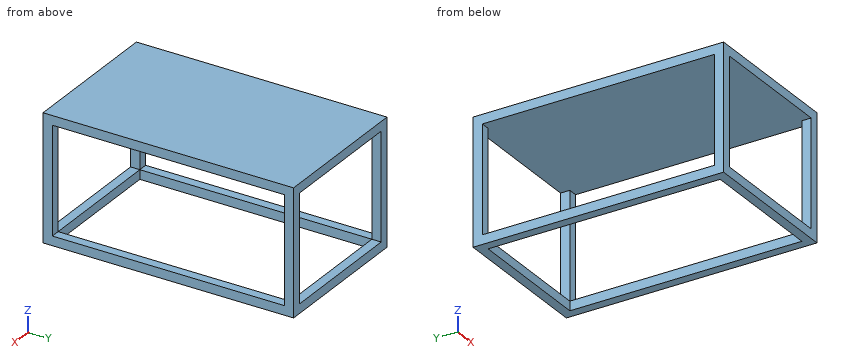
```python
from build123d import *

# Parameters (mm, degrees)
F0_W     = 406.4
F0_H     = 685.8
F1_DEPTH = 25.4
F2_W     = 25.4
F2_H     = 25.4
F3_DEPTH = 317.5
F4_W     = 406.4
F4_H     = 685.8
F5_DEPTH = 25.4
F6_W     = 355.6
F6_H     = 635
F7_DEPTH = 25.4


with BuildPart() as f1:
    # F0 (on Top) → F1 (new body)
    with BuildSketch(Plane.XY):
        Rectangle(F0_W, F0_H)
    extrude(amount=F1_DEPTH)

    # F2 (on face) → F3 (join)
    with BuildSketch(Plane(origin=(0, 0, 0), x_dir=(1, 0, 0), z_dir=(0, 0, -1))):
        with Locations((190.5, 330.2)):
            Rectangle(F2_W, F2_H)
        with Locations((-190.5, -330.2)):
            Rectangle(F2_W, F2_H)
        with Locations((190.5, -330.2)):
            Rectangle(F2_W, F2_H)
        with Locations((-190.5, 330.2)):
            Rectangle(F2_W, F2_H)
    extrude(amount=F3_DEPTH)

    # F4 (on face) → F5 (join)
    with BuildSketch(Plane(origin=(0, 0, -317.5), x_dir=(1, 0, 0), z_dir=(0, 0, -1))):
        Rectangle(F4_W, F4_H)
    extrude(amount=-F5_DEPTH)

    # F6 (on face) → F7 (cut)
    with BuildSketch(Plane(origin=(0, 0, -317.5), x_dir=(1, 0, 0), z_dir=(0, 0, -1))):
        Rectangle(F6_W, F6_H)
    extrude(amount=-F7_DEPTH, mode=Mode.SUBTRACT)


solid = f1.part
```
Model file for the job. Use its own axes, mm. Give positions to 0.01 mm unless a question says otherwise; leave off trailing zeros. Loops run counter-clockwise (first coordinate to the right, second up) from the corner with the lowest first, then second, coordinate; pieces in that order, holes last. Notation, with made-up numbers: (-21.5, 81) -> (14.5, 81) arc R23 ccw to (14.5, 113) -> close; hole circle Ø9 at (42.5, 85). An arc over 180 degrees is marked (long way). Write each question's results on one line, items separated by ' | '.
(1) Probe line 1 along Z through (x, y) = (182, -197.5); line 2 along Z through (x, y) = (75.5, -86). List the from-to ranges inside material, lowest first.
Geometry results:
line 1: z = -317.5 to -292.1, 0 to 25.4 | line 2: z = 0 to 25.4
(2) Cut at C-C on x = -112.5. List the corners of the cut face in (y, z).
Geometry results:
outline: (-342.9, -317.5) -> (-317.5, -317.5) -> (-317.5, -292.1) -> (-342.9, -292.1) -> close; (-342.9, 0) -> (342.9, 0) -> (342.9, 25.4) -> (-342.9, 25.4) -> close; (317.5, -317.5) -> (342.9, -317.5) -> (342.9, -292.1) -> (317.5, -292.1) -> close
(3) Cut at A-A on z = -230.5. List the corners of the cut face in (x, y), and give its area (3 significant figures).
Geometry results:
outline: (-203.2, -342.9) -> (-177.8, -342.9) -> (-177.8, -317.5) -> (-203.2, -317.5) -> close; (-203.2, 317.5) -> (-177.8, 317.5) -> (-177.8, 342.9) -> (-203.2, 342.9) -> close; (177.8, -342.9) -> (203.2, -342.9) -> (203.2, -317.5) -> (177.8, -317.5) -> close; (177.8, 317.5) -> (203.2, 317.5) -> (203.2, 342.9) -> (177.8, 342.9) -> close | area: 2,580 mm²
(4) Cut at B-B on y = 113. List the corners of the cut face in (x, z).
Geometry results:
outline: (-203.2, -317.5) -> (-177.8, -317.5) -> (-177.8, -292.1) -> (-203.2, -292.1) -> close; (-203.2, 0) -> (203.2, 0) -> (203.2, 25.4) -> (-203.2, 25.4) -> close; (177.8, -317.5) -> (203.2, -317.5) -> (203.2, -292.1) -> (177.8, -292.1) -> close
(5) Flat gauge pin, fed straight in: pin 1 Ø3 at (x, y) = (15, 48.5) entering from -Z. Where does the tip first touch, or does it go through?
Geometry results:
pin 1: stops at z = 0
